Check sheet for the modelled part. Datum: model origin and axes. Units: mm. Coordinates: 2 decimals unless noted, no trailing zeros. Write each loop counter-clockwise with the first axis right and the second up, starting at its lowest first coordinate (ties: lowest second). Pieces come first, ordered by that corner, then holes. Notation, with made-up numbers: M 70,9 L 101,9 A17 cw 101,35 Z; hole C 85,-1 d5. An arc over 180 degrees is marked long. Answer as CSV lines item,"result". Start each with the question number.
1) Section check A-A (y = -12). Record the cut outline in (x, z) (3 decimals).
2) Section check C-C (y = -59.5). Record the cut outline in (x, z) (3 decimals).
3) Section check D-D (x = -5). Record the cut outline in (y, z) (3 decimals), and give its area (3 significant figures).
4) Section check B-B (z = 1.2). Record the cut outline in (x, y).
5) Go/stop test with a flat-tipped pin: pin 1 Ø1.6 at (y, z) = (-0.5, 2) entering from -X. Record where the tip stops, or that it passes through.
6) Material ranges on L1, parallel to X at y = -59.5, z = 0.65; L2, parallel to X at y = -29.5, z = 0.9; L3, parallel to Y at x = 10, z = 2.75, recorded low to high. Write a range as [from, to].
Solid Edge part; units mm, degrees
sketch "Sketch1" plane through (0, 0, 0) normal (0, 0, 1) x (1, 0, 0)
  line L0 (-146.05, 139.7) -> (-146.05, -139.7)
  line L1 (-146.05, -139.7) -> (146.05, -139.7)
  line L2 (146.05, -139.7) -> (146.05, 139.7)
  line L3 (146.05, 139.7) -> (-146.05, 139.7)
  dimension "D1" = 146.05
  dimension "D2" = 146.05
extrude "Protrusion1" add sketch "Sketch1" along normal blind 3.175
sketch "Sketch2" plane through (0, 0, 3.175) normal (0, 0, 1) x (1, 0, 0)
  line L0 (-50.8, -139.7) -> (-50.8, 76.2)
  line L1 (-50.8, 76.2) -> (50.8, 76.2)
  line L2 (50.8, 76.2) -> (50.8, -139.7)
  line L3 (50.8, -139.7) -> (-50.8, -139.7)
  dimension "D1" = 50.8
  dimension "D2" = 50.8
extrude "Cutout1" cut sketch "Sketch2" against normal up to next
chamfer "Chamfer_1" distance 19.05 angle 45 2 edges at (-50.8, -139.7, 1.5875) (50.8, -139.7, 1.5875)
sketch "Sketch3" plane through (0, 0, 3.175) normal (0, 0, 1) x (1, 0, 0)
  line L0 (-146.05, 38.1) -> (-146.05, -38.1)
  line L1 (-146.05, -38.1) -> (-127, -38.1)
  line L2 (-127, -38.1) -> (-127, 38.1)
  line L3 (-127, 38.1) -> (-146.05, 38.1)
  dimension "D1" = 127
  dimension "D2" = 127
extrude "Cutout2" cut sketch "Sketch3" against normal up to next
sketch "Sketch4" plane through (0, 0, 3.175) normal (0, 0, 1) x (1, 0, 0)
  line L0 (146.05, 38.1) -> (146.05, -38.1)
  line L1 (146.05, -38.1) -> (127, -38.1)
  line L2 (127, -38.1) -> (127, 38.1)
  line L3 (127, 38.1) -> (146.05, 38.1)
  dimension "D1" = 127
  dimension "D2" = 146.05
extrude "Cutout3" cut sketch "Sketch4" against normal up to next
properties part number "SPaRC-01-005"
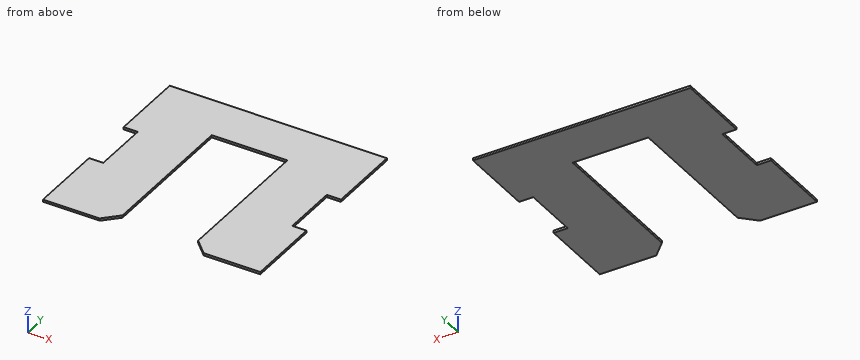
Results found:
1,outline,"M -127,0 L -50.8,0 L -50.8,3.175 L -127,3.175 Z; M 50.8,0 L 127,0 L 127,3.175 L 50.8,3.175 Z"
2,outline,"M -146.05,0 L -50.8,0 L -50.8,3.175 L -146.05,3.175 Z; M 50.8,0 L 146.05,0 L 146.05,3.175 L 50.8,3.175 Z"
3,outline,"M 76.2,0 L 139.7,0 L 139.7,3.175 L 76.2,3.175 Z"
3,area,"202 mm2"
4,outline,"M -146.05,-139.7 L -69.85,-139.7 L -50.8,-120.65 L -50.8,76.2 L 50.8,76.2 L 50.8,-120.65 L 69.85,-139.7 L 146.05,-139.7 L 146.05,-38.1 L 127,-38.1 L 127,38.1 L 146.05,38.1 L 146.05,139.7 L -146.05,139.7 L -146.05,38.1 L -127,38.1 L -127,-38.1 L -146.05,-38.1 Z"
5,pin 1,"stops at x = -127"
6,L1,"x = [-146.05, -50.8], [50.8, 146.05]"
6,L2,"x = [-127, -50.8], [50.8, 127]"
6,L3,"y = [76.2, 139.7]"
